The listing builds one solid part. Answer for the finished solid, in the listing's coordinates (mm). Face numbers are marked on the shaded views. Give positions to 0.01 mm unless a question says otherwise; leave off trailing zeros. Write each loop counter-clockwise with the first axis right and the second up, starting at its lowest first coordinate (ties: lowest second). Pieces come first, ordered by that corner, then holes.
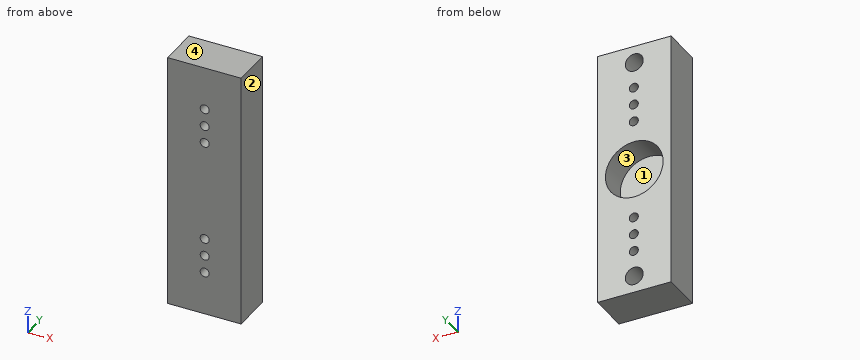
Autodesk Inventor part; units mm, degrees
ref_plane "YZ Plane" through (0, 0, 0) normal (1, 0, 0) x (0, 1, 0)
ref_plane "XZ Plane" through (0, 0, 0) normal (0, 1, 0) x (-1, 0, 0)
ref_plane "XY Plane" through (0, 0, 0) normal (0, 0, 1) x (1, 0, 0)
sketch "Sketch1" plane through (0, 0, 0) normal (0, 1, 0) x (-1, 0, 0)
  line L0 (19.05, -83) -> (19.05, 83)
  line L1 (-19.05, 83) -> (-19.05, -83)
  circle A0 centre (0, 0) radius 11.5094
  line L2 (0, 0) -> (-0.4877, 3.251) construction
  line L3 (0, 0) -> (0, 44.45) construction
  line L4 (0, 0) -> (0, -44.45) construction
  circle A1 centre (0, 44.45) radius 3.5719
  circle A2 centre (0, -44.45) radius 3.5719
  line L5 (19.05, 83) -> (-19.05, 83)
  line L6 (19.05, -83) -> (-19.05, -83)
  dimension "d2" = 23.0188
  dimension "d4" = 44.45
  dimension "d5" = 44.45
  dimension "d6" = 7.1437
  dimension "d7" = 7.1437
extrude "Extrusion1" add sketch "Sketch1" along normal blind 25.4
sketch "Sketch6" plane through (0, 0, 0) normal (0, -1, 0) x (1, 0, 0)
  circle A0 centre (0, 44.45) radius 3.5719
  circle A1 centre (0, 44.45) radius 3.5719
  circle A2 centre (0, -44.45) radius 3.5719
  circle A3 centre (0, -44.45) radius 3.5719
  circle A4 centre (0, 0) radius 5.1594
  circle A5 centre (0, 0) radius 11.5094
  dimension "d102" = 35.7188
sketch "Sketch13" plane through (0, 25.4, 0) normal (0, 1, 0) x (1, 0, 0)
  line L0 (-19.05, -83) -> (19.05, -83) construction
  line L1 (0.1743, -83) -> (0.1743, 83) construction
  line L2 (19.05, 83) -> (-19.05, 83) construction
  circle A0 centre (0.1743, -34) radius 1.8
  circle A1 centre (0.1743, -27) radius 1.8
  circle A2 centre (0.1743, -20) radius 1.8
  circle A3 centre (0.1743, 20) radius 1.8
  circle A4 centre (0.1743, 27) radius 1.8
  circle A5 centre (0.1743, 34) radius 1.8
  circle A6 centre (0, 0) radius 11.5094
  line L3 (-19.05, 83) -> (-19.05, -83)
  line L4 (-19.05, -83) -> (-14.6844, -83)
  line L5 (-14.6844, -83) -> (-14.6844, 83)
  line L6 (-14.6844, 83) -> (-19.05, 83)
  line L7 (-19.05, 83) -> (-19.05, -83)
  line L8 (19.05, -83) -> (14.6844, -83)
  line L9 (14.6844, -83) -> (14.6844, 83)
  line L10 (14.6844, 83) -> (19.05, 83)
  line L11 (19.05, 83) -> (19.05, -83)
  dimension "d82" = 3.6
  dimension "d83" = 3.6
  dimension "d84" = 3.6
  dimension "d85" = 3.6
  dimension "d86" = 3.6
  dimension "d87" = 3.6
  dimension "d88" = 7
  dimension "d89" = 7
  dimension "d90" = 7
  dimension "d92" = 7
  dimension "d93" = 20
  dimension "d94" = 20
  dimension "d97" = 3.175
  dimension "d99" = 3.175
sketch "Sketch14" plane through (19.05, 0, -83) normal (0, 0, -1) x (-1, 0, 0)
  line L0 (0, 0) -> (0, 25.4)
  line L1 (38.1, 0) -> (38.1, 25.4)
  line L2 (0, 25.4) -> (38.1, 25.4)
  line L3 (38.1, 25.4) -> (38.1, 16.2292)
  line L4 (38.1, 16.2292) -> (0, 16.2292)
  line L5 (0, 16.2292) -> (0, 25.4)
  point P0 (19.05, 0)
extrude "Extrusion15" cut sketch "Sketch14" against normal up to next
sketch "Sketch15" plane through (-19.05, 16.2292, -83) normal (0, 1, 0) x (1, 0, 0)
  line L0 (38.1, -166) -> (0, -166)
  line L1 (38.1, 0) -> (38.1, -166)
  line L2 (0, -166) -> (38.1, -166)
  line L3 (38.1, -166) -> (38.1, -134.1969)
  line L4 (38.1, -134.1969) -> (0, -134.1969)
  line L5 (0, -134.1969) -> (0, -166)
  circle A0 centre (19.05, -127.45) radius 3.5719
  line L6 (0, -166) -> (0, 0)
  line L7 (0, 0) -> (38.1, 0)
  line L8 (38.1, 0) -> (38.1, -31.8031)
  line L9 (38.1, -31.8031) -> (0, -31.8031)
  line L10 (0, -31.8031) -> (0, 0)
  circle A1 centre (19.05, -38.55) radius 3.5719
  point P0 (19.05, -83)
  dimension "d78" = 3.175
  dimension "d79" = 3.175
extrude "Extrusion16" cut sketch "Sketch15" against normal up to next contours L0 L5 L4 L1 | L9 L6 L7 L1
extrude "Extrusion18" cut sketch "Sketch13" against normal up to next contours A0 | A1 | A2 | A3 | A4 | A5 | L6 L5 L4 L3 | L8 L9 L10 L11
extrude "Extrusion19" add sketch "Sketch6" against normal blind 5 contours A0 | A2 | A4 | A5
properties part number "RodBase"
Item 1: A cutting plane is placed at A-A, the plane z = 20. Give the vertices of the cut face in (x, y).
Conclusion:
outline: (-14.68, 0) - (-1.63, 0) - (-1.63, 16.23) - (-14.68, 16.23) - close; (1.97, 0) - (14.68, 0) - (14.68, 16.23) - (1.97, 16.23) - close
Item 2: A cutting plane is placed at B-B, the plane y = 13. Count the separate pieces of the cut face and the enclosed holes in it, plus the area to 3 significant figures.
Conclusion:
separate pieces: 1
enclosed holes: 9
area: 2,450 mm2
Item 3: Each of these flat-tipped pins is pushed along its axis until it touches: P1, Ø4, axis at x = 0.17, z = 27, coming from the +Y side; P2, Ø3.5, axis at x = 1, z = -43.5, coming from the +Y side; P3, Ø2, axis at x = 0.17, z = 20, coming from the -Y side. Where does it stop, or does it pass through?
Conclusion:
P1: stops at y = 16.23
P2: stops at y = 5
P3: passes through
Item 4: A cutting plane is placed at C-C, the plane z = -44.45. Give the vertices of the cut face in (x, y), plus the area to 3 significant figures.
Conclusion:
outline: (-14.68, 0) - (14.68, 0) - (14.68, 16.23) - (3.57, 16.23) - (3.57, 5) - (-3.57, 5) - (-3.57, 16.23) - (-14.68, 16.23) - close
area: 396 mm2
Item 5: Determine the mould class of the marked faces 1, 2, 3 and 4 for opening direction Z: pulls with the +Z half, pulls with the -Z half, needs draft (parallel to the pull), parting line crosses it, or undercut.
Conclusion:
face 1: undercut
face 2: needs draft
face 3: undercut
face 4: pulls with the +Z half
Item 6: Consider probe 1 along X at (y, z) = (9.75, -34); probe 2 along Z at (x, y) = (3, 13.5); probe 3 along X at (y, z) = (8.25, -32.5). Determine where each line is inside the solid, lowest interval first.
Conclusion:
probe 1: x = -14.68 to -1.63, 1.97 to 14.68
probe 2: z = -51.2 to -46.39, -42.51 to -11.11, 11.11 to 42.51, 46.39 to 51.2
probe 3: x = -14.68 to -0.82, 1.17 to 14.68
Item 7: A cutting plane is placed at D-D, the plane x = -4.5. Give the vertices of the cut face in (y, z), plus the area to 3 significant figures.
Conclusion:
outline: (0, -51.2) - (16.23, -51.2) - (16.23, -10.59) - (5, -10.59) - (5, 10.59) - (16.23, 10.59) - (16.23, 51.2) - (0, 51.2) - close
area: 1,420 mm2
